```python
from build123d import *

# Parameters (mm, degrees)
SKETCH1_R           = 2
SKETCH1_R_2         = 1.5
BOSS_EXTRUDE1_DEPTH = 1.5
BOSS_EXTRUDE2_DEPTH = 1.5


with BuildPart() as part:
    # Sketch1 → Boss-Extrude1 (new, symmetric)
    # profile 1 of 4: a face of its own
    with BuildSketch(Plane(origin=(0, 0, 0), x_dir=(1, 0, 0), z_dir=(0, 1, 0))):
        with BuildLine():
            Line((-12, 4), (-18, 4))
            ThreePointArc((-18, 4), (-22, 0), (-18, -4))
            Line((-18, -4), (-12, -4))
            Line((-12, -4), (-12, -2))
            Line((-12, -2), (12, -2))
            Line((12, -2), (12, -3))
            Line((12, -3), (18, -3))
            ThreePointArc((18, -3), (21, 0), (18, 3))
            Line((18, 3), (12, 3))
            Line((12, 3), (12, 2))
            Line((12, 2), (-12, 2))
            Line((-12, 2), (-12, 4))
        make_face()
        with Locations(Location((-17.5, 0, 0), (0, 0, 270))):
            Circle(SKETCH1_R, mode=Mode.SUBTRACT)
        with Locations(Location((17.5, 0, 0), (0, 0, 270))):
            Circle(SKETCH1_R_2, mode=Mode.SUBTRACT)
    # profile 2 of 4: a face of its own
    with BuildSketch(Plane(origin=(0, 0, 0), x_dir=(1, 0, 0), z_dir=(0, 1, 0))):
        with BuildLine():
            Line((12, -2), (8.127016654, -2))
            ThreePointArc((8.127016654, -2), (10.127016654, -2.254033308), (12, -3))
            Line((12, -3), (12, -2))
        make_face()
    # profile 3 of 4: a face of its own
    with BuildSketch(Plane(origin=(0, 0, 0), x_dir=(1, 0, 0), z_dir=(0, 1, 0))):
        with BuildLine():
            Line((-12, -2), (-12, -4))
            ThreePointArc((-12, -4), (-9.536924503, -2.516685226), (-6.708497378, -2))
            Line((-6.708497378, -2), (-12, -2))
        make_face()
    # profile 4 of 4: a face of its own
    with BuildSketch(Plane(origin=(0, 0, 0), x_dir=(1, 0, 0), z_dir=(0, 1, 0))):
        with BuildLine():
            Line((-12, 4), (-12, 2))
            Line((-12, 2), (-6.708497378, 2))
            ThreePointArc((-6.708497378, 2), (-9.536924503, 2.516685226), (-12, 4))
        make_face()
    extrude(amount=BOSS_EXTRUDE1_DEPTH, both=True)

    # Sketch2 → Boss-Extrude2 (add, symmetric)
    with BuildSketch(Plane(origin=(0, 0, 0), x_dir=(1, 0, 0), z_dir=(0, 1, 0))):
        with BuildLine():
            Line((8.127016654, 2), (12, 2))
            Line((12, 2), (12, 3))
            ThreePointArc((12, 3), (10.127016654, 2.254033308), (8.127016654, 2))
        make_face()
    extrude(amount=BOSS_EXTRUDE2_DEPTH, both=True)


solid = part.part
```
CAD build for the part. Positions are in the model's coordinates, mm. A direction names the side the tool comes from. Give positions to 0.01 mm unless a question says otherwise; leave off trailing zeros. Order: outer loops, then holes, each group sorted by start corner. A loop starts at its lowest first (then second) coordinate and runs counter-clockwise, first axis right, second up. Notation, with made-up numbers: M -6,-6 L 3,-6 A10 ccw 3,11 Z; hole C 81,62.25 d9. An arc over 180 degrees is marked long. Put each result on its own line as item: value. Start each with the question number.
(1) Saw through at C-C, the plane x = -17.5. Write the cut outline in (y, z), then the cut area to 3 significant figures.
(2) Drill centre lines: line 1 along X through (y, z) = (0.6, 0); line 2 along X through (y, z) = (1.1, -0.5); line 3 along Z through (x, y) = (1, -0.2). Where is each one in solid material? Low to high.
(3) Saw through at B-B, the plane y = 1. Write the cut outline in (x, z).
(4) Flat gauge pins, fed straight in: pin 1 Ø0.9 at (x, y) = (3, 0.5) entering from +Z; pin 2 Ø0.9 at (x, y) = (15.5, 0) entering from +Z; pin 3 Ø0.9 at (x, y) = (-3, -0.5) entering from -Z. Where does each tip first touch, or does it go through?
(5) Saw through at D-D, the plane z = 2.5. Write the cut outline in (x, y).
(6) Which spindle directions (+Z, -Z, +X, -X, +Y, -Y) get a long thin tool onto all of the face, cutting with end or side? Do faces 1 (the flat face through (1, 0, -2)), 2 (the flat face through (15, 0, -3)), 3 (the cylindrical face through (10.1, -0.021, 2.247)), 4 (the flat face through (15, 0, 3)). Say none if no direction does.
(7) Mould opens along Z. For faces 5 (the cylindrical face through (-22, 0, 0)), 6 (the cylindrical face through (-15.517, -0.021, -0.26)), 7 (the cylindrical face through (18.765, -0.021, 0.806)), 8 (the cylindrical face through (-9.499, 0.021, -2.502)) say: +Z half, -Z half, draft (parallel to the pull), parting line (faces both ways), or undercut.
(8) Saw through at A-A, the plane z = 0. Write the cut outline in (x, y).
Check result:
1. outline: M -1.5,-4 L 1.5,-4 L 1.5,-2 L -1.5,-2 Z; M -1.5,2 L 1.5,2 L 1.5,4 L -1.5,4 Z
1. area: 12.0 mm2
2. line 1: x = -22 to -19.5, -15.5 to 16, 19 to 21
2. line 2: x = -21.97 to -19.44, -15.56 to 16.09, 18.91 to 20.96
2. line 3: z = -2 to 2
3. outline: M -18,-4 L -12,-4 A8 cw -6.71,-2 L 8.13,-2 A8 cw 12,-3 L 18,-3 A3 ccw 18,3 L 12,3 A8 cw 8.13,2 L -6.71,2 A8 cw -12,4 L -18,4 A4 ccw Z; hole C -17.5,0 d4; hole C 17.5,0 d3
4. pin 1: stops at z = 2
4. pin 2: stops at z = 3
4. pin 3: stops at z = -2
5. outline: M -21.12,-1.5 L -9.49,-1.5 L -9.49,1.5 L -21.12,1.5 Z; M 10.91,-1.5 L 19.66,-1.5 L 19.66,1.5 L 10.91,1.5 Z
6. face 1: -Z, +Y, -Y
6. face 2: -Z, +X, +Y, -Y
6. face 3: +Z, +Y, -Y
6. face 4: +Z, +X, +Y, -Y
7. face 5: parting line
7. face 6: undercut
7. face 7: undercut
7. face 8: -Z half
8. outline: M -22,-1.5 L -19.5,-1.5 L -19.5,1.5 L -22,1.5 Z; M -15.5,-1.5 L 16,-1.5 L 16,1.5 L -15.5,1.5 Z; M 19,-1.5 L 21,-1.5 L 21,1.5 L 19,1.5 Z
